Autodesk Inventor part; units mm, degrees
ref_plane "YZ Plane" through (0, 0, 0) normal (1, 0, 0) x (0, 1, 0)
ref_plane "XZ Plane" through (0, 0, 0) normal (0, 1, 0) x (-1, 0, 0)
ref_plane "XY Plane" through (0, 0, 0) normal (0, 0, 1) x (1, 0, 0)
sketch "Sketch1" plane through (0, 0, 0) normal (0, 0, 1) x (1, 0, 0)
  line L0 (10, -10) -> (-10, -10)
  line L1 (-10, -10) -> (-10, 10)
  line L2 (-10, 10) -> (10, 10)
  line L3 (10, 10) -> (10, -10)
  circle A0 centre (0, 5) radius 1.2
  circle A1 centre (0, -5) radius 1.2
  circle A2 centre (0, 0) radius 3
  dimension "d0" = 10
  dimension "d1" = 10
  dimension "d2" = 10
  dimension "d3" = 10
  dimension "d4" = 5
  dimension "d5" = 5
  dimension "d6" = 2.4
  dimension "d7" = 2.4
  dimension "d8" = 6
extrude "Extrusion1" add sketch "Sketch1" along normal blind 5
sketch "Sketch2" plane through (0, 0, 5) normal (0, 0, 1) x (1, 0, 0)
  line L0 (0, 0) -> (-1.3346, -1.3533)
  circle A0 centre (6, -6) radius 2.5
  circle A1 centre (6, 6) radius 2.5
  line L1 (10, -10) -> (10, 10)
  line L2 (-10, -10) -> (10, -10)
  line L3 (10, 10) -> (-10, 10)
  dimension "d34" = 4
  dimension "d35" = 4
  dimension "d36" = 4
  dimension "d37" = 4
  dimension "d38" = 5
  dimension "d39" = 5
extrude "Extrusion2" cut sketch "Sketch2" against normal blind 1
sketch "Sketch7" plane through (0, 0, 0) normal (0, 0, -1) x (-1, 0, 0)
  circle A0 centre (-6, 6) radius 2.5
  circle A1 centre (-6, 6) radius 1.375
  circle A2 centre (-6, -6) radius 2.5
  circle A3 centre (-6, -6) radius 1.375
  point P0 (0, 0)
  dimension "d40" = 2.75
  dimension "d41" = 2.75
extrude "Extrusion6" cut sketch "Sketch7" against normal blind 5 contours A1 | A3
sketch "Sketch8" plane through (0, 0, 5) normal (0, 0, 1) x (1, 0, 0)
  line L0 (10, 10) -> (-10, 10)
  line L1 (10, 10) -> (2.5, 10)
  line L2 (2.5, 10) -> (2.5, 2.5)
  line L3 (2.5, 2.5) -> (10, 2.5)
  line L4 (10, 2.5) -> (10, 10)
  line L5 (10, -10) -> (10, 10)
  line L6 (10, -10) -> (2.5, -10)
  line L7 (2.5, -10) -> (2.5, -2.5)
  line L8 (2.5, -2.5) -> (10, -2.5)
  line L9 (10, -2.5) -> (10, -10)
  line L10 (10, -2.5) -> (5, -2.5)
  line L11 (5, -2.5) -> (5, 2.5)
  line L12 (5, 2.5) -> (10, 2.5)
  line L13 (10, 2.5) -> (10, -2.5)
  circle A0 centre (6, 6) radius 2.5
  circle A1 centre (6, 6) radius 2.5
  circle A2 centre (6, -6) radius 2.5
  circle A3 centre (6, -6) radius 2.5
  point P0 (0, 0)
  point P1 (2.5, 10)
  dimension "d44" = 7.5
  dimension "d45" = 7.5
  dimension "d46" = 7.5
  dimension "d47" = 7.5
  dimension "d48" = 5
extrude "Extrusion7" add sketch "Sketch8" along normal blind 5
sketch "Sketch9" plane through (0, 0, 0) normal (0, 0, -1) x (-1, 0, 0)
  circle A0 centre (-6, 6) radius 1.375
  circle A1 centre (-6, 6) radius 2
  circle A2 centre (-6, -6) radius 1.375
  circle A3 centre (-6, -6) radius 2
  point P0 (0, 0)
  dimension "d51" = 4
  dimension "d52" = 4
extrude "Extrusion8" cut sketch "Sketch9" against normal blind 2 contours A0 | A1 | A2 | A3
sketch "Sketch10" plane through (0, 0, 0) normal (0, 0, -1) x (-1, 0, 0)
  line L0 (-2.5, 10) -> (10, 10)
  line L1 (10, -10) -> (-2.5, -10)
  line L2 (10, 10) -> (5, 10)
  line L3 (5, 10) -> (5, -10)
  line L4 (5, -10) -> (10, -10)
  line L5 (10, -10) -> (10, 10)
  line L6 (5, 10) -> (2, 10)
  line L7 (2, 10) -> (2, 5)
  line L8 (2, 5) -> (5, 5)
  line L9 (5, 5) -> (5, 10)
  line L10 (5, -10) -> (2, -10)
  line L11 (2, -10) -> (2, -5)
  line L12 (2, -5) -> (5, -5)
  line L13 (5, -5) -> (5, -10)
  point P0 (0, 0)
  dimension "d55" = 5
  dimension "d56" = 3
  dimension "d57" = 5
  dimension "d58" = 5
  dimension "d59" = 3
extrude "Extrusion9" cut sketch "Sketch10" against normal blind 10
sketch "Sketch11" plane through (-2, 5, 0) normal (-1, 0, 0) x (0, 0, 1)
  circle A0 centre (2.5, 2.5) radius 1.025
  line L0 (0, 5) -> (5, 5)
  line L1 (0, 0) -> (0, 5)
  circle A1 centre (2.5, -12.5) radius 1.025
  line L2 (5, -15) -> (0, -15)
  line L3 (0, -15) -> (0, -10)
  point P0 (0, -5)
  dimension "d62" = 2.5
  dimension "d63" = 2.5
  dimension "d64" = 2.05
  dimension "d65" = 2.5
  dimension "d66" = 2.5
  dimension "d67" = 2.05
extrude "Extrusion10" cut sketch "Sketch11" against normal blind 5
thread "Thread1"
thread "Thread2"
equation "\"d7\" = d6"
equation "\"d39\" = d38"
equation "\"d45\" = d44"
equation "\"d46\" = d45"
equation "\"d52\" = d51"
equation "\"d65\" = d62"
equation "\"d66\" = d63"
equation "\"d67\" = d64"
properties part number "MotorMount"
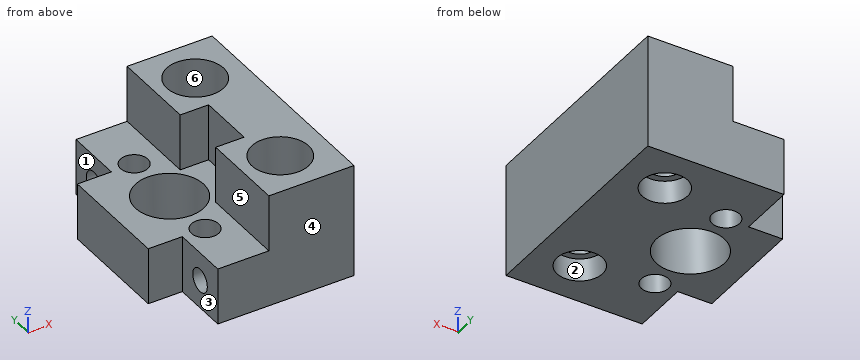
Geometry: final body of the model. Coordinates: model frame, mm. Face numbers are marked on the shaded views. A direction names the side the tool comes from. Coordinates: 2 decimals unless noted, no trailing zeros. Order: outer loops, then holes, each group sorted by start corner. A loop starts at its lowest first (then second) coordinate and runs counter-clockwise, first axis right, second up.
(1) Access query for the marked faces 1, 2 and 3. Directions: +Z, -Z, +X, -X, +Y, -Y. A direction counts if a zero-diameter tool reaches every point of the face in a straight line with its end or side. Return the directions, or none.
(2) Section query A-A (y = 0). Return the cut outline in (x, z), plus the area to 3 significant figures.
(3) Section query B-B (x = -1.5). Return the cut outline in (y, z) (3 decimals), plus the area to 3 significant figures.
(4) Section query C-C (z = 2.5). Return the cut outline in (x, y) (3 decimals), plus the area to 3 significant figures.
(5) First-contact query: pin 1 (6 mm diameter, centred on x = 0.5, z = 8.5, fed in from +Y); pin 2 (2.5 mm diameter, centred on y = -8, z = 3, fed in from -X); pin 3 (3 mm diameter, centred on x = 6, y = 6, fed in from +Z); pin 4 (2 mm diameter, centred on x = 0, y = -5, fed in from -Z). Flat tips, straight axial feed; report the tip coordinate or a pass-through.
(6) Draft query along X for the marked faces 4, 5 and 6. Return one class per face: pulls with the +X half, pulls with the -X half, needs draft (parallel to the pull), parting line crosses it, or undercut.
(7) Material intervals for probe 1 along Y at (x, z) = (6, 6.6); probe 2 along X at (y, z) = (4.5, 9.5); probe 3 along Y at (x, z) = (0.55, 2.5) (3 decimals), sorted ascending.
(8) Section query D-D (z = 7.75). Return the cut outline in (x, y).
Solution:
1. face 1: +Z, -Z, -X, +Y
1. face 2: -Z
1. face 3: +Z, -Z, -X, -Y
2. outline: (-5, 0) - (-3, 0) - (-3, 5) - (-5, 5) - close; (3, 0) - (10, 0) - (10, 10) - (5, 10) - (5, 5) - (3, 5) - close
2. area: 70.0 mm2
3. outline: (-10, 0) - (-2.598, 0) - (-2.598, 5) - (-10, 5) - close; (2.598, 0) - (10, 0) - (10, 5) - (2.598, 5) - close; hole circle Ø2.05 at (-7.5, 2.5); hole circle Ø2.05 at (7.5, 2.5)
3. area: 67.4 mm2
4. outline: (-5, -5) - (-2, -5) - (-2, -6.475) - (3, -6.475) - (3, -8.525) - (-2, -8.525) - (-2, -10) - (10, -10) - (10, 10) - (-2, 10) - (-2, 8.525) - (3, 8.525) - (3, 6.475) - (-2, 6.475) - (-2, 5) - (-5, 5) - close; hole circle Ø6 at (0, 0); hole circle Ø2.4 at (0, -5); hole circle Ø2.4 at (0, 5); hole circle Ø2.75 at (6, -6); hole circle Ø2.75 at (6, 6)
4. area: 200 mm2
5. pin 1: stops at y = 10
5. pin 2: stops at x = -2
5. pin 3: stops at z = 4
5. pin 4: passes through
6. face 4: needs draft
6. face 5: pulls with the -X half
6. face 6: undercut
7. probe 1: y = -10 to -8.5, -3.5 to 3.5, 8.5 to 10
7. probe 2: x = 2.5 to 4, 8 to 10
7. probe 3: y = -10 to -8.525, -6.475 to -6.067, -3.933 to -2.949, 2.949 to 3.933, 6.067 to 6.475, 8.525 to 10
8. outline: (2.5, -10) - (10, -10) - (10, 10) - (2.5, 10) - (2.5, 2.5) - (5, 2.5) - (5, -2.5) - (2.5, -2.5) - close; hole circle Ø5 at (6, -6); hole circle Ø5 at (6, 6)
